Geometry: final body of the model. Coordinates: model frame, mm. Round coordinates to 2 decimals unless told otherwise and drop trailing zeros. Loops run counter-clockwise (first coordinate to the right, second up) from the corner with the lowest first, then second, coordinate; pieces in that order, holes last. Notation, with made-up numbers: M 14.25,65 L 24.25,65 A32 cw 24.25,95 Z; hole C 30.5,80.25 d11. An arc over 180 degrees is marked long. Return JSON: item names as keys, results as strings.
from build123d import *

# Parameters (mm, degrees)
F0_W     = 30
F0_H     = 10
F1_DEPTH = 10
F2_W     = 10
F2_H     = 10
F3_DEPTH = 10
F4_R     = 1.5
F5_DEPTH = 10.001
F7_DEPTH = 10.001


with BuildPart() as f1:
    # F0 (on Top) → F1 (new body)
    with BuildSketch(Plane.XY):
        Rectangle(F0_W, F0_H)
    extrude(amount=F1_DEPTH)

    # F2 (on face) → F3 (join)
    with BuildSketch(Plane.XY.offset(10)):
        Rectangle(F2_W, F2_H)
    extrude(amount=F3_DEPTH)

    # F4 (on face) → F5 (cut, through all)
    with BuildSketch(Plane.XZ.offset(5)):
        with Locations((0, 7.772714)):
            Circle(F4_R)
    extrude(amount=-F5_DEPTH, mode=Mode.SUBTRACT)

    # F6 (on face) → F7 (cut, through all)
    with BuildSketch(Plane.XZ.offset(5)):
        Polygon((-15, 0), (-5, 10), (-15, 10), align=None)
        Polygon((-5, 20), (-5, 10), (0, 20), align=None)
        Polygon((5, 20), (0, 20), (5, 10), align=None)
        Polygon((15, 10), (5, 10), (15, 0), align=None)
    extrude(amount=-F7_DEPTH, mode=Mode.SUBTRACT)


solid = f1.part
Q1. Material intervals for L1, parallel to X at y = 3, z = 6.5; L2, parallel to Z at x = 2.5, y = -3.75; L3, parallel to X at y = -0.5, z = 15, sorted ascending.
Determined:
{"L1": "x = -8.5 to -0.79, 0.79 to 8.5", "L2": "z = 0 to 15", "L3": "x = -2.5 to 2.5"}
Q2. Section query D-D (x = -4). Output: boundary loops of the cut face in (y, z).
Determined:
{"outline": "M -5,0 L 5,0 L 5,12 L -5,12 Z"}
Q3. Section query B-B (z = 7). Output: boundary loops of the cut face in (x, y).
Determined:
{"outline": "M -8,-5 L -1.29,-5 L -1.29,5 L -8,5 Z; M 1.29,-5 L 8,-5 L 8,5 L 1.29,5 Z"}
Q4. Section query A-A (y = 3.25). Output: boundary loops of the cut face in (x, z).
Determined:
{"outline": "M -15,0 L 15,0 L 5,10 L 0,20 L -5,10 Z; hole C 0,7.77 d3"}
Q5. Section query C-C (x = 10). Output: boundary loops of the cut face in (y, z).
Determined:
{"outline": "M -5,0 L 5,0 L 5,5 L -5,5 Z"}
Q6. Pull-direction query (Z, two-part tool) for faces 1 (the cylindrical face through (0.806, -0.07, 9.038)), 2 (the flat face through (0, 0, 0)), 3 (the flat face through (10, 0, 5)); classes: pulls with the +Z half, pulls with the -Z half, needs draft (parallel to the pull), parting line crosses it, or undercut.
Determined:
{"face 1": "undercut", "face 2": "pulls with the -Z half", "face 3": "pulls with the +Z half"}
